```python
from build123d import *

# Parameters (mm, degrees)
PAD025_DEPTH    = 12.6
PAD026_DEPTH    = 10.2
POCKET012_DEPTH = 1
SKETCH058_R     = 2.2
POCKET022_DEPTH = 6
CHAMFER002_SIZE = 0.6


with BuildPart() as part:
    # Sketch039 → Pad025 (new body)
    with BuildSketch(Plane.XY.offset(14.6)):
        with BuildLine():
            Line((-3, -11.5), (3, -11.5))
            ThreePointArc((7, -15.5), (5.828427, -12.671573), (3, -11.5))
            Line((7, -15.5), (7, -23))
            Line((7, -23), (18, -23))
            ThreePointArc((22, -27), (20.828427, -24.171573), (18, -23))
            Line((22, -27), (22, -30.5))
            ThreePointArc((18, -34.5), (20.828427, -33.328427), (22, -30.5))
            Line((18, -34.5), (7, -34.5))
            Line((7, -34.5), (7, -42))
            ThreePointArc((3, -46), (5.828427, -44.828427), (7, -42))
            Line((3, -46), (-3, -46))
            ThreePointArc((-7, -42), (-5.828427, -44.828427), (-3, -46))
            Line((-7, -42), (-7, -34.5))
            Line((-7, -34.5), (-18, -34.5))
            ThreePointArc((-22, -30.5), (-20.828427, -33.328427), (-18, -34.5))
            Line((-22, -30.5), (-22, -27))
            ThreePointArc((-18, -23), (-20.828427, -24.171573), (-22, -27))
            Line((-18, -23), (-7, -23))
            Line((-7, -23), (-7, -15.5))
            ThreePointArc((-3, -11.5), (-5.828427, -12.671573), (-7, -15.5))
        make_face()
    extrude(amount=PAD025_DEPTH)

    # Sketch041 (on Face21 of Pad025) → Pad026 (join)
    with BuildSketch(Plane(origin=(0, 0, 14.6), x_dir=(1, 0, 0), z_dir=(0, 0, -1))):
        Polygon((-17, 36.5), (-9, 36.5), (-9, 41.5), (9, 41.5), (9, 36.5), (17, 36.5), (17, 21), (9, 21), (9, 16), (-9, 16), (-9, 21), (-17, 21), align=None)
    extrude(amount=-PAD026_DEPTH)

    # Sketch042 (on Face5 of Pad026) → Pocket012 (cut)
    with BuildSketch(Plane.XY.offset(27.2)):
        Polygon((0, -16.75), (-2.5, -21.080127), (2.5, -21.080127), align=None)
        Polygon((-2.5, -36.419873), (2.5, -36.419873), (0, -40.75), align=None)
        Polygon((-16.330127, -28.75), (-12, -26.25), (-12, -31.25), align=None)
        Polygon((12, -26.25), (12, -31.25), (16.330127, -28.75), align=None)
    extrude(amount=-POCKET012_DEPTH, mode=Mode.SUBTRACT)

    # Sketch058 (on Face8 of Pocket012) → Pocket022 (cut)
    with BuildSketch(Plane(origin=(0, 0, 14.6), x_dir=(1, 0, 0), z_dir=(0, 0, -1))):
        with Locations((0, 28.75)):
            Circle(SKETCH058_R)
    extrude(amount=-POCKET022_DEPTH, mode=Mode.SUBTRACT)

    # Chamfer002
    chamfer002_edges = [part.edges().sort_by_distance(p)[0] for p in [
        (-14.165064, -30, 27.2),
        (-14.165064, -27.5, 27.2),
        (-12, -28.75, 27.2),
        (12, -28.75, 27.2),
        (0, -11.5, 27.2),
        (-5.828427, -12.671573, 27.2),
        (5.828427, -12.671573, 27.2),
        (-7, -19.25, 27.2),
        (7, -19.25, 27.2),
        (-12.5, -23, 27.2),
        (12.5, -23, 27.2),
        (-20.828427, -24.171573, 27.2),
        (20.828427, -24.171573, 27.2),
        (-22, -28.75, 27.2),
        (22, -28.75, 27.2),
        (-20.828427, -33.328427, 27.2),
        (20.828427, -33.328427, 27.2),
        (-12.5, -34.5, 27.2),
        (12.5, -34.5, 27.2),
        (-7, -38.25, 27.2),
        (7, -38.25, 27.2),
        (-5.828427, -44.828427, 27.2),
        (5.828427, -44.828427, 27.2),
        (0, -46, 27.2),
        (14.165064, -27.5, 27.2),
        (14.165064, -30, 27.2),
        (1.25, -18.915064, 27.2),
        (0, -21.080127, 27.2),
        (-1.25, -18.915064, 27.2),
        (0, -36.419873, 27.2),
        (1.25, -38.584936, 27.2),
        (-1.25, -38.584936, 27.2),
    ]]
    chamfer(chamfer002_edges, length=CHAMFER002_SIZE)


solid = part.part
```
Source: CAD feature listing. Evaluate the final solid. Frame: model axes, mm. A direction names the side the tool comes from. Give positions to 0.01 mm unless a question says otherwise; leave off trailing zeros. Write each loop counter-clockwise with the first axis right and the second up, starting at its lowest first coordinate (ties: lowest second). Pieces come first, ordered by that corner, then holes.
1. Access query for faces 4 (the face through (11, -36, 24.8)), 5 (the face through (-14, -29, 26.2)), 6 (the face through (-13, -36.5, 20)). Directions: +Z, -Z, +X, -X, +Y, -Y. A direction counts if a zero-diameter tool reaches every point of the face in a straight line with its end or side. Return the directions, or none.
2. Pull-direction query (X, two-part tool) for faces 1 (the face through (-9, -39, 20)), 2 (the face through (-14.356, -27.269, 26.896)), 3 (the face through (8, -16, 20)); classes: +X half, -X half, draft (parallel to the pull), parting line (faces both ways), or undercut.
3. Material intervals for line 1 along X through (y, z) = (-29, 26.75); line 2 along Y through (x, z) = (0, 19.25); line 3 along X through (y, z) = (-28.75, 19), sorted ascending.
4. Section query B-B (x = -14). Return the cut outline in (y, z).
5. Section query A-A (x = -7.5). Return the cut outline in (y, z).
6. First-contact query: pin 1 (2 mm diameter, centred on y = -38, z = 20, fed in from +X); pin 2 (1.3 mm diameter, centred on x = 0.5, y = -18.5, fed in from +Z); pin 3 (2 mm diameter, centred on y = -39, z = 22.5, fed in from -X). Flat tips, straight axial feed; report the tip coordinate or a pass-through.
Output values:
1. face 4: +Z, +X, -Y
1. face 5: +Z
1. face 6: +Z, -Z, -X, -Y
2. face 1: -X half
2. face 2: undercut
2. face 3: draft
3. line 1: x = -21.85 to -16.2, -11.85 to 11.85, 16.2 to 21.85
3. line 2: y = -46 to -30.95, -26.55 to -11.5
3. line 3: x = -22 to -2.2, 2.2 to 22
4. outline: (-36.5, 14.6) - (-21, 14.6) - (-21, 24.8) - (-23, 24.8) - (-23, 26.6) - (-23.6, 27.2) - (-26.71, 27.2) - (-27.4, 26.6) - (-27.4, 26.2) - (-30.1, 26.2) - (-30.1, 26.6) - (-30.79, 27.2) - (-33.9, 27.2) - (-34.5, 26.6) - (-34.5, 24.8) - (-36.5, 24.8) - close
5. outline: (-41.5, 14.6) - (-16, 14.6) - (-16, 24.8) - (-23, 24.8) - (-23, 26.6) - (-23.6, 27.2) - (-33.9, 27.2) - (-34.5, 26.6) - (-34.5, 24.8) - (-41.5, 24.8) - close
6. pin 1: stops at x = 9
6. pin 2: stops at z = 26.81
6. pin 3: stops at x = -9
